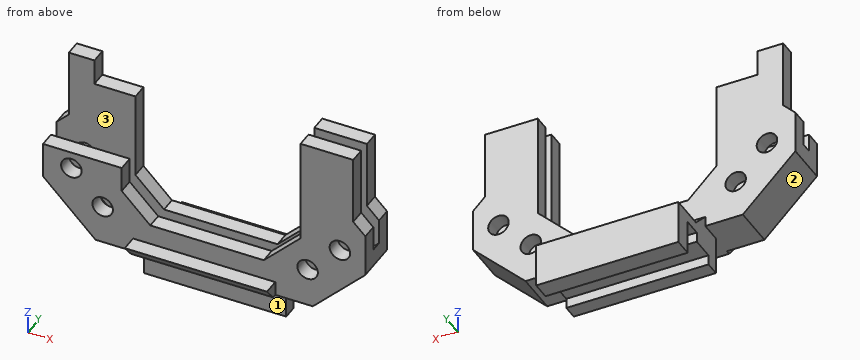
Autodesk Inventor part; units mm, degrees
ref_plane "Work Plane1" through (59.9208, 47.0911, 21.911) normal (0, 1, 0) x (-1, 0, 0)
ref_plane "Work Plane2" through (59.9208, 45.8611, 21.911) normal (0, -1, 0) x (1, 0, 0)
ref_plane "Work Plane13" through (59.9208, 43.8611, -18.7491) normal (1, 0, 0) x (0, 0, -1)
ref_plane "Work Plane1" through (59.9208, 47.0911, 21.911) normal (0, 1, 0) x (-1, 0, 0)
sketch "Sketch1" plane through (59.9208, 47.0911, 21.911) normal (0, 1, 0) x (-1, 0, 0)
  circle A0 centre (-16.808, -43.6345) radius 1.27
  circle A1 centre (12.5729, -47.6345) radius 1.27
  circle A2 centre (16.4459, -43.6345) radius 1.27
  circle A3 centre (-12.808, -47.6345) radius 1.27
  line L0 (10.208, -33.8805) -> (10.208, -44.6601)
  line L1 (10.208, -44.6601) -> (6.6725, -48.1956)
  circle A4 centre (-16.808, -43.6345) radius 1.27
  circle A5 centre (12.5729, -47.6345) radius 1.27
  circle A6 centre (16.4459, -43.6345) radius 1.27
  circle A7 centre (-12.8081, -47.6345) radius 1.27
  line L2 (19.708, -15.6655) -> (-19.708, -15.6655)
  line L3 (0, -15.6655) -> (0, -20.8781)
  line L4 (6.6725, -48.1956) -> (-7.3796, -48.1956)
  line L5 (-19.958, -43.8381) -> (-12.8316, -50.9645)
  line L6 (-12.8316, -50.9645) -> (12.8316, -50.9645)
  line L7 (-19.958, -40.6601) -> (-19.958, -43.8381)
  line L8 (0, -48.1956) -> (0, -46.7038)
  line L9 (19.958, -43.8381) -> (12.8316, -50.9645)
  line L10 (19.958, -40.6601) -> (19.958, -43.8381)
  line L11 (-11.938, -30.6601) -> (-11.938, -43.6372)
  line L12 (-10.5616, -45.0137) -> (-11.938, -43.6372)
  line L13 (-10.5616, -45.0137) -> (-7.3796, -48.1956)
  line L14 (15.2967, -30.6601) -> (18.458, -30.6601)
  line L15 (18.458, -30.6601) -> (18.458, -39.1601)
  line L16 (-18.458, -39.1601) -> (-18.458, -30.6601)
  line L17 (-18.458, -30.6601) -> (-11.938, -30.6601)
  line L18 (10.208, -33.8805) -> (15.2967, -33.8805)
  line L19 (15.2967, -33.8805) -> (15.2967, -30.6601)
  line L20 (-19.958, -40.6601) -> (-18.458, -39.1601)
  line L21 (19.958, -40.6601) -> (18.458, -39.1601)
  point P0 (-19.708, -43.6601)
  point P1 (-6.6725, -48.1956)
  dimension "d14" = 5
  dimension "d15" = 135
  dimension "d18" = 2.54
extrude "Extrusion1" add sketch "Sketch1" along normal blind 2
ref_plane "Work Plane2" through (59.9208, 45.8611, 21.911) normal (0, -1, 0) x (1, 0, 0)
sketch "Sketch2" plane through (59.9208, 45.8611, 21.911) normal (0, -1, 0) x (1, 0, 0)
  line L0 (-10.208, -33.8805) -> (-10.208, -44.6601)
  line L1 (-10.208, -44.6601) -> (-6.6725, -48.1956)
  line L2 (-6.6725, -48.1956) -> (7.3796, -48.1956)
  circle A0 centre (16.808, -43.6345) radius 1.27
  circle A1 centre (-12.5729, -47.6345) radius 1.27
  circle A2 centre (-16.4459, -43.6345) radius 1.27
  circle A3 centre (12.808, -47.6345) radius 1.27
  line L3 (19.958, -40.6601) -> (19.958, -43.8381)
  line L4 (19.958, -43.8381) -> (12.8316, -50.9645)
  line L5 (12.8316, -50.9645) -> (-12.8316, -50.9645)
  line L6 (-12.8316, -50.9645) -> (-19.958, -43.8381)
  line L7 (-19.958, -43.8381) -> (-19.958, -40.6601)
  line L8 (7.3796, -48.1956) -> (11.938, -43.6372)
  line L9 (11.938, -43.6372) -> (11.938, -30.6601)
  line L10 (11.938, -30.6601) -> (18.458, -30.6601)
  line L11 (18.458, -30.6601) -> (18.458, -39.1601)
  line L12 (-18.458, -39.1601) -> (-18.458, -30.6601)
  line L13 (-18.458, -30.6601) -> (-15.2967, -30.6601)
  line L14 (-15.2967, -30.6601) -> (-15.2967, -33.8805)
  line L15 (-15.2967, -33.8805) -> (-10.208, -33.8805)
  line L16 (18.458, -39.1601) -> (19.958, -40.6601)
  line L17 (-19.958, -40.6601) -> (-18.458, -39.1601)
  circle A4 centre (-16.4459, -43.6345) radius 1.27
  line L18 (-19.958, -43.8381) -> (-19.958, -40.6601)
  line L19 (-19.958, -41.5123) -> (-10.208, -41.5123)
  line L20 (-10.208, -33.8805) -> (-10.208, -44.6601)
  point P0 (-59.9208, -21.911)
extrude "Extrusion2" add sketch "Sketch2" along normal blind 2 contours L0 L1 L2 L8 L9 L10 L11 L16 L3 L4 L5 L6 L7 L19
sketch "Sketch4" plane through (79.8789, 45.8611, -18.7491) normal (1, 0, 0) x (0, 0, -1)
  line L0 (0, 1.23) -> (3.178, 1.23)
  line L1 (0, 0) -> (-1.5, 0)
  line L2 (0, 1.23) -> (0, 0)
  line L3 (-12.1065, -0.085) -> (12.1065, -0.085)
  line L4 (12.1065, -0.085) -> (12.1065, 1.315)
  line L5 (12.1065, 1.315) -> (-12.1065, 1.315)
  line L6 (-12.1065, 1.315) -> (-12.1065, -0.085)
  line L7 (-12.1065, -0.085) -> (12.1065, 1.315) construction
  line L8 (12.1065, -0.085) -> (-12.1065, 1.315) construction
  point P0 (0, 0.615)
  dimension "d73" = 1.4
extrude "Extrusion3" cut sketch "Sketch4" against normal through all
sketch "Sketch5" plane through (59.9208, 43.8611, 21.911) normal (0, -1, 0) x (1, 0, 0)
  line L0 (-19.708, -43.6601) -> (-19.708, -40.6601)
  line L1 (-12.6424, -50.7145) -> (-19.708, -43.6601)
  line L2 (12.728, -50.7145) -> (-12.6424, -50.7145)
  line L3 (19.708, -43.7345) -> (12.728, -50.7145)
  line L4 (-13.4529, -52.4645) -> (13.4529, -52.4645)
  line L5 (19.708, -43.7345) -> (19.708, -40.6601)
  line L6 (-12.8316, -50.9145) -> (12.8316, -50.9145)
  line L7 (12.8316, -50.9645) -> (11.3316, -52.4645)
  line L8 (-19.958, -43.8381) -> (-12.8316, -50.9645)
  line L9 (-12.8316, -50.9645) -> (-11.3316, -52.4645)
  line L10 (-12.8316, -50.9645) -> (-10.7103, -50.9645) construction
  line L11 (12.8316, -50.9145) -> (12.8816, -50.9145)
  line L12 (-12.8316, -50.9645) -> (12.8316, -50.9645)
  line L13 (12.8316, -50.9645) -> (12.8816, -50.9145)
  line L14 (12.8316, -50.9645) -> (19.958, -43.8381)
  line L15 (-12.8316, -50.9145) -> (-12.8816, -50.9145)
  line L16 (-12.8316, -50.9645) -> (-12.8816, -50.9145)
  line L17 (12.8109, -50.9145) -> (19.958, -43.7673)
  line L18 (-19.958, -43.7673) -> (-12.8109, -50.9145)
  line L19 (-19.958, -45.9594) -> (-13.4529, -52.4645)
  line L20 (13.4529, -52.4645) -> (19.958, -45.9594)
  line L21 (-19.958, -43.7673) -> (-19.958, -45.9594)
  line L22 (12.8316, -50.9645) -> (19.958, -43.8381)
  line L23 (19.958, -43.8381) -> (19.958, -45.9594)
  line L24 (19.958, -43.8381) -> (19.958, -43.7673)
  line L25 (19.958, -43.8381) -> (19.958, -40.6601)
  dimension "d29" = 0.2
  dimension "d62" = 45
  dimension "d74" = 0.05
  dimension "d75" = 0.05
  dimension "d76" = 1.5
  dimension "d77" = 1.5
extrude "Extrusion4" add sketch "Sketch5" against normal up to surface (5.23 mm away)
ref_plane "Work Plane13" through (59.9208, 43.8611, -18.7491) normal (1, 0, 0) x (0, 0, -1)
ref_plane "Work Plane14" through (53.2483, 46.4761, -26.2847) normal (0, 1, 0) x (1, 0, 0)
sketch "Sketch18" plane through (59.9208, 43.8611, -18.7491) normal (1, 0, 0) x (0, 0, -1)
  line L0 (12.8044, 2.651) -> (16.5534, 2.651)
  line L1 (16.5534, 2.651) -> (16.5534, 4.4515)
  line L2 (16.5534, 4.4515) -> (15.3033, 4.4515)
  line L3 (15.3033, 4.4515) -> (15.3033, 7.2794)
  line L4 (15.3033, 7.2794) -> (14.0544, 7.2794)
  line L5 (14.0544, 7.2794) -> (14.0544, 9.48)
  line L6 (14.0544, 9.48) -> (18.2804, 9.48)
  line L7 (18.2804, 9.48) -> (18.2804, 11.73)
  line L8 (18.2804, 11.73) -> (12.8044, 11.73)
  line L9 (12.8044, 7.48) -> (12.8044, 11.73)
  line L10 (12.8044, 2.651) -> (11.8044, 2.651)
  line L11 (11.8044, 0) -> (10.0544, 0)
  line L12 (10.0544, 0) -> (10.0544, -2)
  line L13 (10.0544, -2) -> (11.8044, -0.5316)
  line L14 (11.8044, -0.5316) -> (11.8044, 0)
  line L15 (11.8044, 0) -> (11.8044, 5.23)
  line L16 (11.8044, 2.651) -> (11.8044, 5.23)
  line L17 (10.5544, 5.23) -> (12.8044, 7.48)
  line L18 (10.5544, 5.23) -> (11.8044, 5.23)
  point P0 (12.8044, 6.23)
  dimension "d184" = 1.75
  dimension "d185" = 2
  dimension "d186" = 50
extrude "Extrusion12" add sketch "Sketch18" along normal blind 8.804 and the other way blind 8.804
ref_plane "Work Plane19" through (51.1168, 53.1911, -37.0296) normal (0, -1, 0) x (1, 0, 0)
ref_plane "Work Plane20" through (68.7248, 51.1406, -34.2524) normal (0, 0, -1) x (-1, 0, 0)
properties part number "Button Holder"
Part model, mm, in its own coordinate system. Face numbers are marked on the shaded views. A direction names the side the tool comes from. Round coordinates to 2 decimals unless told otherwise and drop trailing zeros. Write each loop counter-clockwise with the first axis right and the second up, starting at its lowest first coordinate (ties: lowest second). Pieces come first, ordered by that corner, then holes. Notation, with made-up numbers: M 62,19 L 70,19 A23 ccw 70,47 Z; hole C 0,52 d6. An arc over 180 degrees is marked long. Answer as CSV lines item,"result". Start each with the question number.
1) Drill centre lines: L1, parallel to Y at x = 65, z = -34.25; L2, parallel to X at y = 44.25, z = -22 (3 decimals); L3, parallel to Y at x = 78, z = -13. Where is each one in solid material? Low to high.
2) Which spindle directions (+Z, -Z, +X, -X, +Y, -Y) get a long thin tool onto all of the face, cutting with end or side? Do the marked faces 1, 2 and 3. Say none if no direction does.
3) Band-saw the part on C-C (y = 45.25). List the corners of the cut face in (x, z), then the cut area to 3 significant figures.
4) Drop flat-ended pins along their axis: pin 1 (1.3 mm diameter, centred on x = 59, y = 53.5, fed in from +Z); pin 2 (2 mm diameter, centred on x = 47.5, y = 48, fed in from +Z); pin 3 (10 mm diameter, centred on x = 56, z = -16.5, fed in from -Y); pin 4 (1.4 mm diameter, centred on x = 58, z = -33.5, fed in from -Y). Give the stop position or say it passes through.
5) Band-saw the part on A-A (z = -34.75). List the corners of the cut face in (x, y).
6) Band-saw the part on B-B (x = 44). List the corners of the cut face in (y, z).
7) Band-saw the part on D-D (z = -14.75). List the corners of the cut face in (x, y), then the cut area to 3 significant figures.
Worked out:
1,L1,"46.51 to 48.31, 53.34 to 55.59"
1,L2,"39.963 to 42.235, 44.714 to 49.713, 71.585 to 75.489, 77.968 to 79.879"
1,L3,"43.86 to 45.78, 47.18 to 49.09"
2,face 1,"-Z, +X, -X, -Y"
2,face 2,"-Z, -X, +Y, -Y"
2,face 3,"+Z"
3,outline,"M 39.96,-24.05 L 46.47,-30.55 L 73.37,-30.55 L 79.88,-24.05 L 79.88,-18.75 L 78.38,-17.25 L 78.38,-8.75 L 71.86,-8.75 L 71.86,-21.73 L 67.3,-26.28 L 53.25,-26.28 L 49.71,-22.75 L 49.71,-19.6 L 39.96,-19.6 Z; hole C 43.47,-21.72 d2.54; hole C 47.35,-25.72 d2.54; hole C 72.73,-25.72 d2.54; hole C 76.73,-21.72 d2.54"
3,area,"316 mm²"
4,pin 1,"z = -31.55"
4,pin 2,"z = -11.97"
4,pin 3,"through"
4,pin 4,"y = 46.51"
5,outline,"M 51.12,46.51 L 68.72,46.51 L 68.72,48.31 L 51.12,48.31 Z; M 51.12,53.34 L 68.72,53.34 L 68.72,55.59 L 51.12,55.59 Z"
6,outline,"M 43.86,-28.09 L 49.09,-28.09 L 49.09,-22.88 L 47.18,-22.88 L 47.18,-25.89 L 45.78,-25.89 L 45.78,-22.88 L 43.86,-22.88 Z; M 43.86,-20.57 L 45.78,-20.57 L 45.78,-19.6 L 43.86,-19.6 Z; M 47.18,-20.57 L 49.09,-20.57 L 49.09,-8.75 L 47.18,-8.75 Z"
7,outline,"M 41.46,47.18 L 49.71,47.18 L 49.71,49.09 L 41.46,49.09 Z; M 71.86,43.86 L 78.38,43.86 L 78.38,45.78 L 71.86,45.78 Z; M 71.86,47.18 L 78.38,47.18 L 78.38,49.09 L 71.86,49.09 Z"
7,area,"40.8 mm²"
